Can you work these out from the model? Positions are in its coordinate system, mm. A direction names the side the tool comes from. Round coordinates to 2 decimals unless told otherwise and drop trailing zeros. Loops run counter-clockwise (first coordinate to the right, second up) from the corner with the lowest first, then second, coordinate; pieces in that order, holes last. Notation, with made-up numbers: (-13.5, -29) -> (8.5, -29) arc R11 cw to (8.5, -19) -> close; hole circle Ø9 at (62, -1.5). An arc over 180 degrees is marked (long way). Write each question's results on one line, items separated by ' | '.
from build123d import *

# Parameters (mm, degrees)
SKETCH1_W           = 142.5
SKETCH1_H           = 94
BOSS_EXTRUDE1_DEPTH = 15
SKETCH2_W           = 126.5
SKETCH2_H           = 78
CUT_EXTRUDE2_DEPTH  = 3
SKETCH3_R           = 2.5
CUT_EXTRUDE3_DEPTH  = 172.368754445
CHAMFER1_SIZE       = 2
SKETCH4_R           = 2.5
CUT_EXTRUDE6_DEPTH  = 172.368754445
SKETCH6_R           = 2.5
CUT_EXTRUDE7_DEPTH  = 172.368754445
SKETCH7_R           = 2.5
CUT_EXTRUDE8_DEPTH  = 5


with BuildPart() as part:
    # Sketch1 → Boss-Extrude1 (new body)
    with BuildSketch(Plane(origin=(0, 0, 0), x_dir=(1, 0, 0), z_dir=(0, 1, 0))):
        with Locations((71.25, 47)):
            Rectangle(SKETCH1_W, SKETCH1_H)
    extrude(amount=BOSS_EXTRUDE1_DEPTH)

    # Sketch2 → Cut-Extrude2 (cut)
    with BuildSketch(Plane(origin=(0, 15, 0), x_dir=(1, 0, 0), z_dir=(0, 1, 0))):
        Polygon((134.5, 92), (8, 92), (8, 94), (2, 94), (2, 0), (8, 0), (8, 2), (134.5, 2), (134.5, 0), (140.5, 0), (140.5, 94), (134.5, 94), align=None)
        with Locations((71.25, 47)):
            Rectangle(SKETCH2_W, SKETCH2_H, mode=Mode.SUBTRACT)
    extrude(amount=-CUT_EXTRUDE2_DEPTH, mode=Mode.SUBTRACT)

    # Sketch3 → Cut-Extrude3 (cut, through all)
    with BuildSketch(Plane(origin=(0, 15, 0), x_dir=(1, 0, 0), z_dir=(0, 1, 0))):
        with Locations(Location((9.65, 47, 0), (0, 0, 270))):
            Circle(SKETCH3_R)
        with Locations(Location((132.85, 47, 0), (0, 0, 270))):
            Circle(SKETCH3_R)
    extrude(amount=-CUT_EXTRUDE3_DEPTH, mode=Mode.SUBTRACT)

    # Chamfer1
    chamfer1_edges = [part.edges().sort_by_distance(p)[0] for p in [
        (0, 7.5, 0),
        (0, 7.5, -94),
        (142.5, 7.5, -94),
        (142.5, 7.5, 0),
    ]]
    chamfer(chamfer1_edges, length=CHAMFER1_SIZE - 0.0001)  # a hair under: the kernel refuses the full size

    # Sketch4 → Cut-Extrude6 (cut, through all)
    with BuildSketch(Plane(origin=(0, 15, 0), x_dir=(1, 0, 0), z_dir=(0, 1, 0))):
        with Locations(Location((50, 79, 0), (0, 0, 270))):
            Circle(SKETCH4_R)
        with Locations(Location((92.5, 79, 0), (0, 0, 270))):
            Circle(SKETCH4_R)
        with Locations(Location((50, 15, 0), (0, 0, 270))):
            Circle(SKETCH4_R)
        with Locations(Location((92.5, 15, 0), (0, 0, 270))):
            Circle(SKETCH4_R)
    extrude(amount=-CUT_EXTRUDE6_DEPTH, mode=Mode.SUBTRACT)

    # Sketch6 → Cut-Extrude7 (cut, through all)
    with BuildSketch(Plane(origin=(0, 15, 0), x_dir=(1, 0, 0), z_dir=(0, 1, 0))):
        with Locations(Location((124.5, 75, 0), (0, 0, 270))):
            Circle(SKETCH6_R)
        with Locations(Location((18, 75, 0), (0, 0, 270))):
            Circle(SKETCH6_R)
        with Locations(Location((18, 19, 0), (0, 0, 270))):
            Circle(SKETCH6_R)
        with Locations(Location((124.5, 19, 0), (0, 0, 270))):
            Circle(SKETCH6_R)
    extrude(amount=-CUT_EXTRUDE7_DEPTH, mode=Mode.SUBTRACT)

    # Sketch7 → Cut-Extrude8 (cut)
    with BuildSketch(Plane.XY):
        with Locations((58.75, 7.646221832)):
            Circle(SKETCH7_R)
        with Locations((83.75, 7.646221832)):
            Circle(SKETCH7_R)
    extrude(amount=-CUT_EXTRUDE8_DEPTH, mode=Mode.SUBTRACT)


solid = part.part
1. If we section it at B-B (z = -47): List the corners of the cut face in (x, y) for me.
Final values:
outline: (0, 0) -> (7.15, 0) -> (7.15, 12) -> (2, 12) -> (2, 15) -> (0, 15) -> close; (12.15, 0) -> (130.35, 0) -> (130.35, 15) -> (12.15, 15) -> close; (135.35, 0) -> (142.5, 0) -> (142.5, 15) -> (140.5, 15) -> (140.5, 12) -> (135.35, 12) -> close
2. If we section it at C-C (x = 124.5): List the corners of the cut face in (y, z) for me.
Final values:
outline: (0, -94) -> (15, -94) -> (15, -92) -> (12, -92) -> (12, -86) -> (15, -86) -> (15, -77.5) -> (0, -77.5) -> close; (0, -72.5) -> (15, -72.5) -> (15, -21.5) -> (0, -21.5) -> close; (0, -16.5) -> (15, -16.5) -> (15, -8) -> (12, -8) -> (12, -2) -> (15, -2) -> (15, 0) -> (0, 0) -> close
3. Please list where these lines run through material, in increasing order: line 1 (X direction, y = 12.75, z = -19); line 2 (Z direction, x = 101, y = 14.5); line 3 (X direction, y = 10.5, z = -79). Write a range as from..to.
Final values:
line 1: 0..2, 8..15.5, 20.5..122, 127..134.5, 140.5..142.5 | line 2: -94..-92, -86..-8, -2..0 | line 3: 0..47.5, 52.5..90, 95..142.5
4. On a 3-axis mill with a long thin cutter (end or side, diameter ignored), from which of +Z, -Z, +X, -X, +Y, -Y can I reach the whole of each face in a straight line? I mean faces 4 (the face through (70, 14, -2)), 5 (the face through (84, 8, -5)), 6 (the face through (51.69, 7.6, -16.84)), 7 (the face through (2, 14, -48)). Say none if no direction works.
Final values:
face 4: +Y | face 5: +Z | face 6: +Y, -Y | face 7: +Z, -Z, +Y
5. If we section it at D-D (x = 83.75): List the corners of the cut face in (y, z) for me.
Final values:
outline: (0, -94) -> (15, -94) -> (15, -92) -> (12, -92) -> (12, -86) -> (15, -86) -> (15, -8) -> (12, -8) -> (12, -2) -> (15, -2) -> (15, 0) -> (10.15, 0) -> (10.15, -5) -> (5.15, -5) -> (5.15, 0) -> (0, 0) -> close
6. We'd pull the mould along Z, two halves only. Please class faces 1 (the face through (134.5, 14, -26)), 2 (the face through (59, 8, -5)), 3 (the face through (95, 8, -79)): pulls with the +Z half, pulls with the -Z half, needs draft (parallel to the pull), parting line crosses it, or undercut.
Final values:
face 1: needs draft | face 2: pulls with the +Z half | face 3: undercut
7. Will these pins go through, and if not, where does the flat tip stop? pin 1 (0.6 mm diameter, centred on y = 13, z = -93, fed in from +X); pin 2 (4 mm diameter, centred on x = 83.75, y = 7.65, fed in from +Z).
Final values:
pin 1: x = 141.8 | pin 2: z = -5
8. If we section it at A-A (x = 9.65): List the corners of the cut face in (y, z) for me, then the cut area to 3 significant figures.
Final values:
outline: (0, -94) -> (15, -94) -> (15, -92) -> (12, -92) -> (12, -86) -> (15, -86) -> (15, -49.5) -> (0, -49.5) -> close; (0, -44.5) -> (15, -44.5) -> (15, -8) -> (12, -8) -> (12, -2) -> (15, -2) -> (15, 0) -> (0, 0) -> close | area: 1,300 mm2
